from build123d import *

# Parameters (mm, degrees)
STOCK_TEST_FINGER_MICHELLE_V2_1_START = -21.07817965
STOCK_TEST_FINGER_MICHELLE_V2_1_DEPTH = 2.5
CUT_EXTRUDE1_START                    = -1.5
SKETCH1_R                             = 1.75
CUT_EXTRUDE1_DEPTH                    = 1.5


# Read off the part's stored shape, not the designer's step: Stock-test_finger_michelle_V2-1
with BuildPart() as part:
    # Stock-test_finger_michelle_V2-1 outline → Stock-test_finger_michelle_V2-1 (new body)
    with BuildSketch(Plane.YZ.offset(STOCK_TEST_FINGER_MICHELLE_V2_1_START)):
        Polygon((0, -6.34419618), (9.2, -15.54419618), (12.7, -15.54419618), (12.7, 18.45580382), (9.2, 18.45580382), (0, 9.25580382), align=None)
    extrude(amount=STOCK_TEST_FINGER_MICHELLE_V2_1_DEPTH)

    # Sketch1 → Cut-Extrude1 (cut)
    with BuildSketch(Plane.ZY.offset(21.07817965).offset(CUT_EXTRUDE1_START)):
        with Locations(Location((-12.29419618, 9.2, 0), (0, 0, 180))):
            Circle(SKETCH1_R)
        with Locations(Location((15.20580382, 9.2, 0), (0, 0, 180))):
            Circle(SKETCH1_R)
    extrude(amount=CUT_EXTRUDE1_DEPTH, mode=Mode.SUBTRACT)


solid = part.part
Source: CAD feature listing. Evaluate the final solid. Frame: model axes, mm. A direction names the side the tool comes from. Give positions to 0.01 mm unless a question says otherwise; leave off trailing zeros. Write each loop counter-clockwise with the first axis right and the second up, starting at its lowest first coordinate (ties: lowest second). Pieces come first, ordered by that corner, then holes. Notation, with made-up numbers: (-30, 54.5) -> (8, 54.5) arc R9 cw to (8, 68.5) -> close; hole circle Ø3 at (-0.75, -11.75). An arc over 180 degrees is marked (long way). Write item = value, one per line.
Q1. Line query: line 1 (Z direction, x = -20.5, y = 9.2); line 2 (X direction, y = 10, z = 14.5); line 3 (Y direction, x = -19.9, z = 13). Output: solid intervals per line, ascending. Write a range as from..to.
Here are the results:
line_1 = -15.54..-14.04, -10.54..13.46, 16.96..18.46
line_2 = -19.58..-18.58
line_3 = 3.74..12.7
Q2. Mould query, pull axis Y, two halves, no side actions, for faces 3 (the face through (-19.578, 9, -12)), 4 (the face through (-21.078, 6, 2)), 5 (the face through (-19.578, 9, 15)), 6 (the face through (-19.846, 4.536, -10.88)). Classes: +Y half, -Y half, draft (parallel to the pull), parting line (faces both ways), or undercut.
Here are the results:
face_3 = undercut
face_4 = draft
face_5 = undercut
face_6 = -Y half
Q3. Cut plane D-D on y = 4. Return loops of the section in (x, z).
Here are the results:
outline = (-21.08, -10.34) -> (-18.58, -10.34) -> (-18.58, 13.26) -> (-21.08, 13.26) -> close
Q4. Cut plane B-B on y = 7.75. Return loops of the section in (x, z), then the cut area to 3 significant figures.
Here are the results:
outline = (-21.08, -14.09) -> (-18.58, -14.09) -> (-18.58, 17.01) -> (-21.08, 17.01) -> (-21.08, 16.19) -> (-19.58, 16.19) -> (-19.58, 14.23) -> (-21.08, 14.23) -> (-21.08, -11.31) -> (-19.58, -11.31) -> (-19.58, -13.27) -> (-21.08, -13.27) -> close
area = 71.9 mm²
Q5. First-contact query: pin 1 (2 mm diameter, centred on y = 9.2, z = 15.21, fed in from -X). Flat tip, straight axial feed; report the tip coordinate or a pass-through.
Here are the results:
pin_1 = -19.58
Q6. Cut plane A-A on x = -19.95. Return loops of the section in (y, z), then the cut area to 3 significant figures.
Here are the results:
outline = (0, -6.34) -> (9.2, -15.54) -> (12.7, -15.54) -> (12.7, 18.46) -> (9.2, 18.46) -> (0, 9.26) -> close; hole circle Ø3.5 at (9.2, -12.29); hole circle Ø3.5 at (9.2, 15.21)
area = 328 mm²
Q7. Cut plane C-C on z = 11. Return loops of the section in (x, y).
Here are the results:
outline = (-21.08, 1.74) -> (-18.58, 1.74) -> (-18.58, 12.7) -> (-21.08, 12.7) -> close
Q8. Reachability of faces 1 (the face through (-20, 0, 2)), 2 (the face through (-20.32, 8.02, 16.5)) from +Z, -Z, +X, -X, +Y, -Y: full face, straight path, thin tool, end or side. Return the list, or none.
Here are the results:
face_1 = +Z, -Z, +X, -X, -Y
face_2 = -X
